Design review of the part built by this model. Coordinates are the model's own, in mm. Face numbers are marked on the shaded views. A direction names the side the tool comes from. Coordinates: 2 decimals unless noted, no trailing zeros. Loops run counter-clockwise (first coordinate to the right, second up) from the corner with the lowest first, then second, coordinate; pieces in that order, holes last. Notation, with made-up numbers: (16.25, 0.5) -> (66.25, 0.5) arc R23 ccw to (66.25, 22.5) -> close; hole circle Ø3 at (44.5, 61). An arc over 180 degrees is marked (long way). Use CSV: the item, a comma, the result in double quotes.
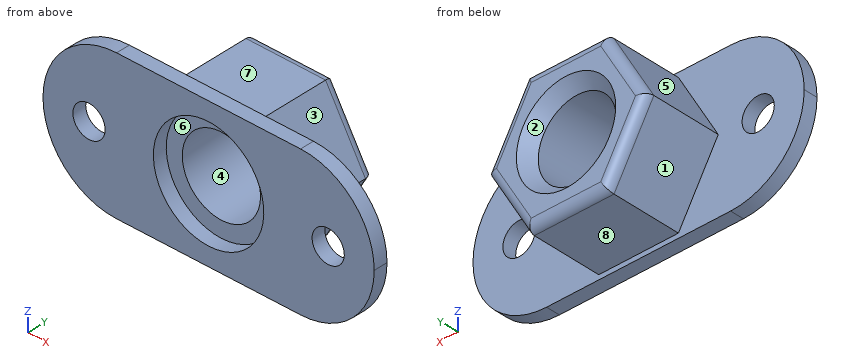
```python
from build123d import *

# Parameters (mm, degrees)
BOSS_EXTRUDE1_DEPTH               = 13.49375
F_5_8_11_TAPPED_HOLE1_D           = 13.49248
F_5_8_11_TAPPED_HOLE1_CSINK_D     = 17.145
F_5_8_11_TAPPED_HOLE1_CSINK_ANGLE = 82
FILLET1_R                         = 1.524
SKETCH4_W                         = 57.15
SKETCH4_H                         = 25.4
BOSS_EXTRUDE2_DEPTH               = 2.38125
FILLET2_R                         = 12.7
SKETCH5_R                         = 9.525
CUT_EXTRUDE1_DEPTH                = 2.38125
SKETCH6_R                         = 2.778125
CUT_EXTRUDE2_DEPTH                = 36.06902123


with BuildPart() as part:
    # Sketch1 → Boss-Extrude1 (new body)
    with BuildSketch(Plane(origin=(0, 0, 0), x_dir=(1, 0, 0), z_dir=(0, 1, 0))):
        Polygon((13.748153285, 0), (6.874076643, 11.90625), (-6.874076643, 11.90625), (-13.748153285, 0), (-6.874076643, -11.90625), (6.874076643, -11.90625), align=None)
    extrude(amount=BOSS_EXTRUDE1_DEPTH)

    # 5/8-11 Tapped Hole1 (through all)
    with Locations(Plane(origin=(0, 13.49375, 0), x_dir=(1, 0, 0), z_dir=(0, 1, 0))):
        with Locations((0, 0)):
            CounterSinkHole(F_5_8_11_TAPPED_HOLE1_D / 2, F_5_8_11_TAPPED_HOLE1_CSINK_D / 2, counter_sink_angle=F_5_8_11_TAPPED_HOLE1_CSINK_ANGLE)

    # Fillet1
    fillet1_edges = [part.edges().sort_by_distance(p)[0] for p in [
        (0, 13.49375, -11.90625),
        (-10.311114964, 13.49375, -5.953125),
        (-10.311114964, 13.49375, 5.953125),
        (0, 13.49375, 11.90625),
        (10.311114964, 13.49375, 5.953125),
        (10.311114964, 13.49375, -5.953125),
    ]]
    fillet(fillet1_edges, radius=FILLET1_R)

    # Sketch4 → Boss-Extrude2 (add)
    with BuildSketch(Plane.XZ):
        Rectangle(SKETCH4_W, SKETCH4_H)
    extrude(amount=BOSS_EXTRUDE2_DEPTH)

    # Fillet2
    fillet2_edges = [part.edges().sort_by_distance(p)[0] for p in [
        (-28.575, -1.190625, -12.7),
        (-28.575, -1.190625, 12.7),
        (28.575, -1.190625, -12.7),
        (28.575, -1.190625, 12.7),
    ]]
    fillet(fillet2_edges, radius=FILLET2_R - 0.0001)  # a hair under: the kernel refuses the full size

    # Sketch5 → Cut-Extrude1 (cut)
    with BuildSketch(Plane.XZ.offset(2.38125)):
        with Locations(Location((0, 0, 0), (0, 0, 270))):
            Circle(SKETCH5_R)
    extrude(amount=-CUT_EXTRUDE1_DEPTH, mode=Mode.SUBTRACT)

    # Sketch6 → Cut-Extrude2 (cut, through all)
    with BuildSketch(Plane.XZ.offset(2.38125)):
        with Locations(Location((-20.6375, 0, 0), (0, 0, 270))):
            Circle(SKETCH6_R)
        with Locations(Location((20.6375, 0, 0), (0, 0, 270))):
            Circle(SKETCH6_R)
    extrude(amount=-CUT_EXTRUDE2_DEPTH, mode=Mode.SUBTRACT)


solid = part.part
```
Item 1: Add section C-C (z = -1). State how many separate pieces and enclosed holes the cut face has, then the cut area to 3 significant figures.
Checked values:
separate pieces,"4"
enclosed holes,"0"
area,"236 mm^2"
Item 2: Draft analysis for pull direction X (two halves, no side actions). For the marked faces 1, 2, 3 and 4, state which applies: pulls with the +X half, pulls with the -X half, needs draft (parallel to the pull), parting line crosses it, or undercut.
Checked values:
face 1,"pulls with the -X half"
face 2,"undercut"
face 3,"pulls with the +X half"
face 4,"undercut"
Item 3: Add section A-A (x = 0). Give the boundary of the cut face in (y, z) (1 decimal).
Checked values:
outline,"(-2.4, -12.7) -> (0, -12.7) -> (0, -11.9) -> (12, -11.9) arc R1.5 ccw to (13.5, -10.4) -> (13.5, -8.6) -> (11.4, -6.7) -> (0, -6.7) -> (0, -9.5) -> (-2.4, -9.5) -> close; (-2.4, 9.5) -> (0, 9.5) -> (0, 6.7) -> (11.4, 6.7) -> (13.5, 8.6) -> (13.5, 10.4) arc R1.5 ccw to (12, 11.9) -> (0, 11.9) -> (0, 12.7) -> (-2.4, 12.7) -> close"
Item 4: Machinability: for the marked faces 5, 6, 7 and 8, which of the approach directions +Z, -Z, +X, -X, +Y, -Y give a long, thin tool a straight path to every point of the face, cutting with its end or side? Answer none if there is none.
Checked values:
face 5,"+Z, -X, +Y"
face 6,"-Y"
face 7,"+Z, +X, -X, +Y"
face 8,"-Z, +X, -X, +Y"
Item 5: Clearance check with flat-ended pins moving along their axes: pin 1 (1.5 mm diameter, centred on x = 3, y = 11.5, fed in from +Z); pin 2 (5 mm diameter, centred on x = 16, z = -4.5, fed in from +Y); pin 3 (5 mm diameter, centred on x = -21.5, y = -0.5, fed in from +Z). State where each tip first meets the part, or that it passes through.
Checked values:
pin 1,"z = 11.91"
pin 2,"y = 0"
pin 3,"z = 12.31"
Item 6: Add section B-B (y = 4.5). Give the boundary of the cut face in (x, z).
Checked values:
outline,"(-13.75, 0) -> (-6.87, -11.91) -> (6.87, -11.91) -> (13.75, 0) -> (6.87, 11.91) -> (-6.87, 11.91) -> close; hole circle Ø13.49 at (0, 0)"
Item 7: Add section D-D (x = -24). Give the boundary of the cut face in (y, z), then the cut area to 3 significant figures.
Checked values:
outline,"(-2.38, -9.76) -> (0, -9.76) -> (0, 9.76) -> (-2.38, 9.76) -> close"
area,"46.5 mm^2"
Item 8: To check wall thickness, follow line 1 along X through (y, z) = (-0.85, 0) (3 decimals); line 2 along Z through (x, y) = (0, 3); line 3 along Y through (x, z) = (-13, 7). State the ranges of each line that lie inside material, in increasing order.
Checked values:
line 1,"-28.575 to -23.416, -17.859 to -9.525, 9.525 to 17.859, 23.416 to 28.575"
line 2,"-11.91 to -6.75, 6.75 to 11.91"
line 3,"-2.38 to 0"
